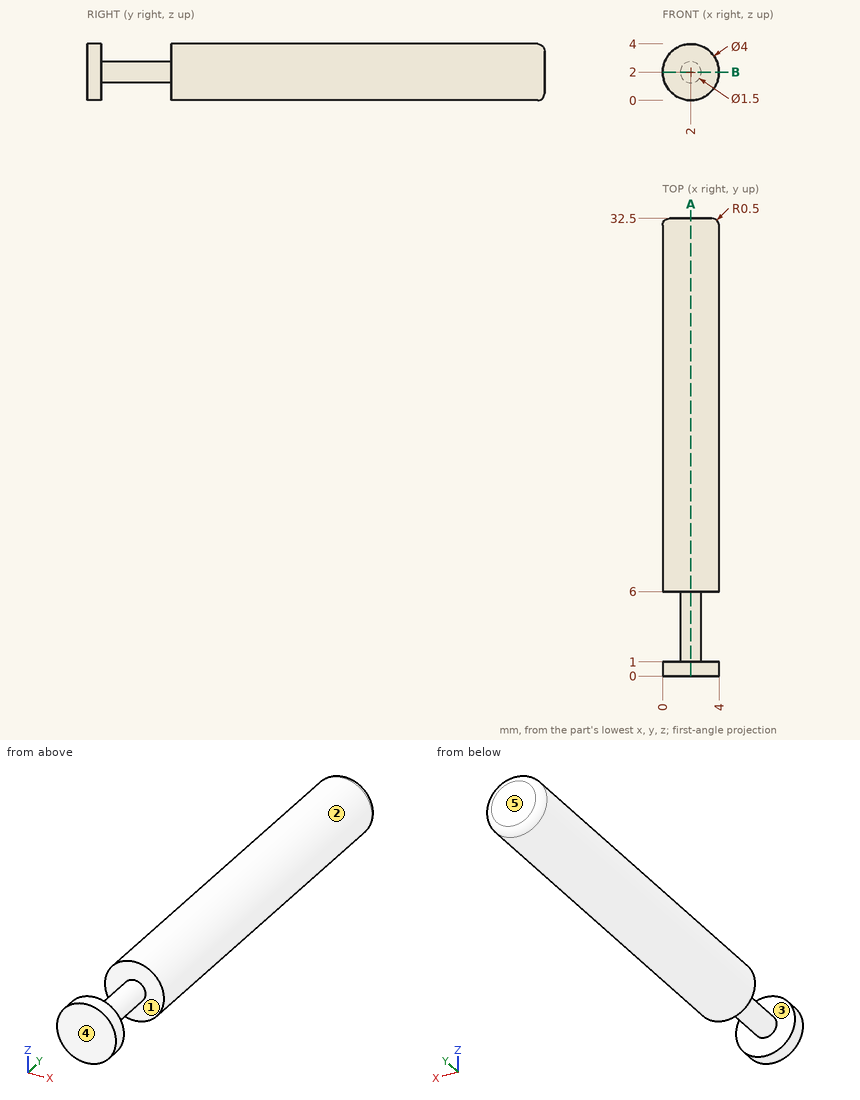
Drawing for the job (mm, zero at the part's lowest x, y, z). A direction names the side the tool comes from. Give positions to 0.01 mm unless a question says otherwise; leave off trailing zeros. Write each loop counter-clockwise with the first axis right and the second up, starting at its lowest first coordinate (ties: lowest second). Pieces come first, ordered by that corner, then holes. Notation, with made-up numbers: (-15, 11) -> (7, 11) arc R18 cw to (7, 34) -> close; hole circle Ø5 at (76, -37.75). An arc over 180 degrees is marked (long way). Put each result on its own line as item: value. Start each with the question number.
Item 1: Wall check: L1, parallel to Y at x = 3.1, z = 2.3; L2, parallel to Z at x = 1.9, y = 28; L3, parallel to Y at x = 3.7, z = 1.1. Give the ranges that are in metal, low to high. Write a range as [from, to].
Item 2: Pin check, flat tip, straight feed: pin 1 Ø1.5 at (x, y) = (2.5, 10) entering from +Z. Stop position of the tip, or through.
Item 3: Which spindle directions (+Z, -Z, +X, -X, +Y, -Y) get a long thin tool onto all of the face, cutting with end or side? Do the marked faces 1 and 2. Say none if no direction does.
Item 4: Cut at A-A (x = 2). List the corners of the cut face in (y, z), then the cut area to 3 significant figures.
Item 5: Pull direction Y, two halves, no side cores. Call the marked faces 3, 4 and 5: pulls with the +Y half, pulls with the -Y half, needs draft (parallel to the pull), parting line crosses it, or undercut.
Item 6: Cut at B-B (z = 2). List the corners of the cut face in (x, y).
Answer list:
1. L1: y = [0, 1], [6, 32.5]
1. L2: z = [0, 4]
1. L3: y = [0, 1], [6, 32.27]
2. pin 1: stops at z = 4
3. face 1: none
3. face 2: +Y, -Y
4. outline: (0, 0) -> (1, 0) -> (1, 1.25) -> (6, 1.25) -> (6, 0) -> (32, 0) arc R0.5 ccw to (32.5, 0.5) -> (32.5, 3.5) arc R0.5 ccw to (32, 4) -> (6, 4) -> (6, 2.75) -> (1, 2.75) -> (1, 4) -> (0, 4) -> close
4. area: 117 mm2
5. face 3: undercut
5. face 4: pulls with the -Y half
5. face 5: pulls with the +Y half
6. outline: (0, 0) -> (4, 0) -> (4, 1) -> (2.75, 1) -> (2.75, 6) -> (4, 6) -> (4, 32) arc R0.5 ccw to (3.5, 32.5) -> (0.5, 32.5) arc R0.5 ccw to (0, 32) -> (0, 6) -> (1.25, 6) -> (1.25, 1) -> (0, 1) -> close
